Work out the finished part from the listing and answer in its coordinate system (mm). Face numbers are marked on the shaded views. A direction names the side the tool comes from. Coordinates: 2 decimals unless noted, no trailing zeros. Order: outer loops, then holes, each group sorted by start corner. A loop starts at its lowest first (then second) coordinate and runs counter-clockwise, first axis right, second up. Notation, with made-up numbers: (64, 15) - (122, 15) arc R30 cw to (122, 53) - close; hole circle Ø6 at (22, 60.25). An arc over 180 degrees is marked (long way). Answer as a JSON object with one key per item and string values. Group by question number.
1) This flat-tipped pin is pushed along its axis until it touches: P1, Ø9.5, axis at x = 39.5, z = 7, coming from the +Y side (3 decimals). Where does it stop, or does it pass through?
2) A tool of negligible diameter and unlimited length cuts with its end or side. For the marked faces 5, 6, 7 and 8, from which of +Z, -Z, +X, -X, +Y, -Y can it reach the whole face along a straight path? Write none if from no direction.
3) Section B-B (x = 34.5) is taken. Give the vertices of the cut face in (y, z) (3 decimals).
4) Section A-A (z = 8.25) is taken. Give the vertices of the cut face in (x, y) (3 decimals), plus the area to 3 significant figures.
5) Find the intervals of material crossed by line 1 along Z through (x, y) = (-45.5, 14); line 2 along Y through (x, z) = (-46, 12) (3 decimals); line 3 along X through (y, z) = (-10, 17.5), in increasing order.
6) The mould has two halves that part along X. Classify the marked faces 1, 2, 3 and 4: released by +X, released by -X, zero draft, split by the parting line, or undercut.
7) Section C-C (x = -19.5) is taken. Give the vertices of the cut face in (y, z).
from build123d import *

# Parameters (mm, degrees)
F1_DEPTH = 19.05
F2_W     = 101.6
F2_H     = 27.813
F3_DEPTH = 6.35
F4_R     = 3.175


with BuildPart() as f1:
    # F0 (on Top) → F1 (new body)
    with BuildSketch(Plane.XY):
        with BuildLine():
            Line((-50.8, -12.7), (50.8, -12.7))
            Line((50.8, -12.7), (50.8, 9.525))
            Line((50.8, 9.525), (23.089258, 9.525))
            ThreePointArc((23.089258, 9.525), (22.605387, 9.351654), (22.341666, 8.910484))
            ThreePointArc((22.341666, 8.910484), (19.37408, 6.353422), (16.182151, 8.624264))
            Line((16.182151, 8.624264), (15.998242, 9.428533))
            ThreePointArc((15.998242, 9.428533), (15.288748, 10.725007), (13.977624, 11.407049))
            ThreePointArc((13.977624, 11.407049), (-0.000865, 12.7), (-13.979325, 11.406732))
            ThreePointArc((-13.979325, 11.406732), (-15.308897, 10.706393), (-16.009978, 9.377212))
            Line((-16.009978, 9.377212), (-16.182151, 8.624264))
            ThreePointArc((-16.182151, 8.624264), (-19.37408, 6.353422), (-22.341666, 8.910484))
            ThreePointArc((-22.341666, 8.910484), (-22.605387, 9.351654), (-23.089258, 9.525))
            Line((-23.089258, 9.525), (-50.8, 9.525))
            Line((-50.8, 9.525), (-50.8, -12.7))
        make_face()
    extrude(amount=F1_DEPTH)

    # F2 (on face) → F3 (join)
    with BuildSketch(Plane(origin=(0, 0, 0), x_dir=(1, 0, 0), z_dir=(0, 0, -1))):
        with Locations((0, -1.2065)):
            Rectangle(F2_W, F2_H)
    extrude(amount=F3_DEPTH)

    # F4
    f4_edges = [f1.edges().sort_by_distance(p)[0] for p in [
        (50.8, 9.525, 9.525),
        (-50.8, 9.525, 9.525),
        (-50.8, -12.7, 6.35),
        (50.8, -12.7, 6.35),
    ]]
    fillet(f4_edges, radius=F4_R)


solid = f1.part
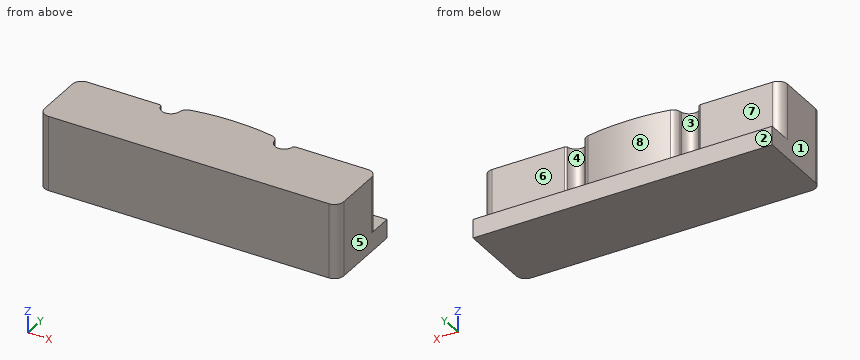
Report:
{
 "1": {"P1": "stops at y = 9.525"},
 "2": {"face 5": "+Z, -Z, +X, +Y, -Y", "face 6": "+Z, +X, +Y", "face 7": "+Z, -X, +Y", "face 8": "+Z, +Y"},
 "3": {"outline": "(-12.7, -6.35) - (15.113, -6.35) - (15.113, 0) - (9.525, 0) - (9.525, 19.05) - (-12.7, 19.05) - close"},
 "4": {"outline": "(-50.8, -9.525) arc R3.175 ccw to (-47.625, -12.7) - (47.625, -12.7) arc R3.175 ccw to (50.8, -9.525) - (50.8, 6.35) arc R3.175 ccw to (47.625, 9.525) - (23.089, 9.525) arc R0.762 ccw to (22.342, 8.91) arc R3.175 cw to (16.182, 8.624) - (15.998, 9.429) arc R2.54 ccw to (13.978, 11.407) arc R76.2 ccw to (-13.979, 11.407) arc R2.54 ccw to (-16.01, 9.377) - (-16.182, 8.624) arc R3.175 cw to (-22.342, 8.91) arc R0.762 ccw to (-23.089, 9.525) - (-47.625, 9.525) arc R3.175 ccw to (-50.8, 6.35) - close", "area": "2,300 mm²"},
 "5": {"line 1": "z = -6.35 to 0", "line 2": "y = -12.7 to 9.525", "line 3": "x = -50.76 to 50.76"},
 "6": {"face 1": "released by -X", "face 2": "zero draft", "face 3": "undercut", "face 4": "undercut"},
 "7": {"outline": "(-12.7, -6.35) - (15.11, -6.35) - (15.11, 0) - (6.36, 0) - (6.36, 19.05) - (-12.7, 19.05) - close"}
}
